Work out the finished part from the listing and answer in its coordinate system (mm). A direction names the side the tool comes from. Round coordinates to 2 decimals unless told otherwise and drop trailing zeros. Loops run counter-clockwise (first coordinate to the right, second up) from the corner with the lowest first, then second, coordinate; pieces in that order, holes last.
```python
from build123d import *

# Parameters (mm, degrees)
EXTRUDE1_DEPTH     = 150
SKETCH2_W          = 49.298496038
SKETCH2_H          = 32.135315936
SKETCH2_W_2        = 47.837799858
CUT_EXTRUDE1_DEPTH = 150
SKETCH3_W          = 134.99868738
SKETCH3_H          = 27.09229113
CUT_EXTRUDE2_DEPTH = 20


with BuildPart() as part:
    # Sketch1 → Extrude1 (new body)
    with BuildSketch(Plane.XY):
        Polygon((-118.530936898, -6.633049378), (-123.315790789, -1.210214968), (-131.077887101, 1.235377021), (-139.690624105, 2.617668145), (-150.429962839, 2.617668145), (-157.235088373, 1.022716848), (-164.571864339, -1.529205227), (-172.440290738, -4.506447648), (-174.566892467, -8.334330761), (-176.055513678, -13.438174912), (-186.582192239, -13.438174912), (-186.582192239, -10.354602404), (-184.880910855, -10.354602404), (-184.880910855, 4.106289356), (-182.966969299, 6.020230912), (-171.802310219, 9.529123766), (-158.83003967, 12.825356447), (-144.794468256, 16.440579387), (-127.462664161, 20.055802326), (-112.895442315, 22.607724402), (-99.391521333, 24.627996045), (-86.121526623, 25.776360974), (-82.676431684, 25.776360974), (-79.231336746, 61.248079229), (-77.827779548, 65.58634693), (-74.765472936, 68.648653542), (58.700056904, 68.648653542), (68.142168958, 66.351923583), (170.984632679, 30.497417), (173.488753661, 27.243716225), (173.664150964, 16.206652811), (173.664150964, -18.244296574), (152.355600789, -18.244296574), (145.337814803, -7.143435106), (138.702817143, -0.508437446), (127.857147893, 2.809061383), (115.480325336, 2.809061383), (101.317157255, 2.809061383), (86.771200848, -0.508437446), (81.284568168, -3.315551841), (78.222261556, -9.312568956), (62.783132387, -38.787270097), (43.133331627, -45.489442613), (-81.740726979, -45.549861026), (-98.221890382, -45.549861026), align=None)
    extrude(amount=EXTRUDE1_DEPTH)

    # Sketch2 → Cut-Extrude1 (cut)
    with BuildSketch(Plane.XY.offset(150)):
        with Locations((-43.524186177, 41.676254948)):
            Rectangle(SKETCH2_W, SKETCH2_H)
        with Locations((20.38127165, 41.676254948)):
            Rectangle(SKETCH2_W_2, SKETCH2_H)
    extrude(amount=-CUT_EXTRUDE1_DEPTH, mode=Mode.SUBTRACT)

    # Sketch3 → Cut-Extrude2 (cut)
    with BuildSketch(Plane(origin=(-84.383919497, 8.195560527, 0), x_dir=(0, 0, 1), z_dir=(-0.995316735, 0.096667453, 0))):
        with Locations((74.261219998, 35.654596801)):
            Rectangle(SKETCH3_W, SKETCH3_H)
    extrude(amount=-CUT_EXTRUDE2_DEPTH, mode=Mode.SUBTRACT)


solid = part.part
```
1. Find section C-C (x = -59.5). Write down the section's boundary in (y, z).
Answer key:
outline: (-45.54, 0) - (25.61, 0) - (25.61, 150) - (-45.54, 150) - close; (57.74, 0) - (68.65, 0) - (68.65, 150) - (57.74, 150) - close
2. Consider probe 1 along Y at (x, z) = (15, 107.5); probe 2 along X at (y, z) = (-9, 83.5); probe 3 along X at (y, z) = (-10, 79.5). Determine where each line is inside the solid, lowest interval first.
Answer key:
probe 1: y = -45.5 to 25.61, 57.74 to 68.65
probe 2: x = -184.88 to -174.76, -117.3 to 78.38, 146.51 to 173.66
probe 3: x = -184.88 to -175.05, -116.77 to 77.86, 147.14 to 173.66
3. Given pin 1 (12 mm diameter, centred on y = 36, z = 128.5, fed in from +X); pin 2 (6 mm diameter, centred on y = 47, z = 78, fed in from -X); pin 3 (0.5 mm diameter, centred on x = -186, z = 39, fed in from +Y), each flat-ended and moving along its own axis, determine where each tip first touches the part or whether it passes through.
Answer key:
pin 1: stops at x = 171.37
pin 2: stops at x = -18.87
pin 3: stops at y = -10.35
4. Find section B-B (y = 37). Write down the section's boundary in (x, z).
Answer key:
outline: (-81.59, 0) - (-68.17, 0) - (-68.17, 6.76) - (-81.59, 6.76) - close; (-81.59, 141.76) - (-68.17, 141.76) - (-68.17, 150) - (-81.59, 150) - close; (-18.87, 0) - (-3.54, 0) - (-3.54, 150) - (-18.87, 150) - close; (44.3, 0) - (152.33, 0) - (152.33, 150) - (44.3, 150) - close
5. Find section D-D (y = -28.5). Write down the section's boundary in (x, z), then the cut area to 3 significant figures.
Answer key:
outline: (-107.12, 0) - (68.17, 0) - (68.17, 150) - (-107.12, 150) - close
area: 26,300 mm2
6. Find section A-A (x = 12.5). Write down the section's boundary in (y, z), then the cut area to 3 significant figures.
Answer key:
outline: (-45.5, 0) - (25.61, 0) - (25.61, 150) - (-45.5, 150) - close; (57.74, 0) - (68.65, 0) - (68.65, 150) - (57.74, 150) - close
area: 12,300 mm2
7. Determine the mould class of faces 4 (the face through (53.1, -42.09, 73.95)), 5 (the face through (-160.852, -0.235, 73.95)), 6 (the face through (-165.407, 11.154, 73.95)) for opening direction X: +X half, -X half, draft (parallel to the pull), parting line (faces both ways), or undercut.
Answer key:
face 4: +X half
face 5: undercut
face 6: -X half
8. Which of the six approach directions +Z, -Z, +X, -X, +Y, -Y give full straight-line access (tool end or side, diameter ignored) to faces 1 (the face through (-73.981, 56.617, 73.316)), 2 (the face through (-153.785, 1.831, 73.95)), 3 (the face through (20, 25.609, 76))?
Answer key:
face 1: -X
face 2: +Z, -Z, -Y
face 3: +Z, -Z
